The listing builds one solid part. Answer for the finished solid, in the listing's coordinates (mm). A direction names the side the tool comes from. Coordinates: 2 decimals unless noted, no trailing zeros. Order: outer loops, then holes, each group sorted by start corner. A loop starts at its lowest first (then second) coordinate and runs counter-clockwise, first axis right, second up. Notation, with made-up numbers: (21.5, -11.5) -> (62.5, -11.5) arc R11 cw to (62.5, -6.5) -> close; hole circle Ø11 at (68, 71). An arc over 180 degrees is marked (long way). Write each question's results on one line, items separated by ' | '. Start each with the question number.
(1) The part is cut by section C-C, the plane y = -32.5. Give the vertices of the cut face in (x, z), then the cut area to 3 significant figures.
(2) The part is cut by section A-A, the plane y = -14. Give the vertices of the cut face in (x, z).
(3) Determine the mould class of faces 5 (the face through (-7, -50.8, 1)), 6 (the face through (-7, -25, -14.924)), 7 (the face through (-7, -12.471, 28)), 8 (the face through (-7, -7, 39.58)) for opening direction Y: +Y half, -Y half, draft (parallel to the pull), parting line (faces both ways), or undercut.
(4) The part is cut by section D-D, the plane x = -31.5. Give the vertices of the cut face in (y, z), then the cut area to 3 significant figures.
(5) Given pin 1 (10.5 mm diameter, centred on x = -11, y = -33, fed in from +Z); pin 2 (20.5 mm diameter, centred on x = 13.5, z = 31, fed in from -Y), each flat-ended and moving along its own axis, determine where each tip first touches the part or whether it passes through.
(6) A tool of negligible diameter and unlimited length cuts with its end or side. For faces 1 (the face through (-6, -48.26, 2)), 2 (the face through (-49.942, -21, 7)), 3 (the face through (-7, -7, 42.12)), 4 (the face through (-7, -49, 16.72)), from which of +Z, -Z, +X, -X, +Y, -Y can it reach the whole face along a straight path? Write none if from no direction.
(7) The part is cut by section B-B, the plane z = 36. Give the vertices of the cut face in (x, y).
(8) Straight lines are drawn through the part: L1, parallel to Y at x = 11, z = 3.5; L2, parallel to Z at x = -32, y = -12; L3, parallel to Y at x = 7.5, z = 37. For each, find the intervals that lie inside material, in ascending order.
```python
from build123d import *

# Parameters (mm, degrees)
F0_W     = 109.3384288251
F0_H     = 31.6438265145
F1_DEPTH = 50.8
F2_W     = 109.3384288251
F2_H     = 15.0109836832
F3_DEPTH = 25.4
F4_DEPTH = 17.78
F5_T     = -2.54


# Not quite as in the source:
# - a shell that OpenCascade refuses in one call is made with other operations: the cavity is built on its own and cut out


with BuildPart() as f1:
    # F0 (on Front) → F1 (new body)
    with BuildSketch(Plane.XZ):
        with Locations((2.1867696196, 0.8977539837)):
            Rectangle(F0_W, F0_H)
    extrude(amount=F1_DEPTH)

    # F2 (on face) → F3 (join)
    with BuildSketch(Plane.XY.offset(16.719667241)):
        with Locations((2.1867696196, -7.5054918416)):
            Rectangle(F2_W, F2_H)
    extrude(amount=F3_DEPTH)

    # F4 (cut): a face of the model
    f4_faces = [f1.faces().sort_by_distance(p)[0] for p in [
        (56.8559840322, -21.9693633853, 6.3658182119),
    ]]
    extrude(f4_faces, amount=-F4_DEPTH, mode=Mode.SUBTRACT)

    # F5: a shell. OpenCascade refuses it in one call, so the cavity is built on its own and cut out:
    # the body offset inwards by the wall thickness, plus a prism from it out through each open face.
    f5_core = offset(f1.part, amount=F5_T, kind=Kind.INTERSECTION, mode=Mode.PRIVATE)
    f5_exits = [f5_core.faces().sort_by_distance(p)[0] for p in [
        (-6.70323, -30.365492, 14.179667),
    ]]
    add(f5_core, mode=Mode.SUBTRACT)
    extrude(f5_exits, amount=-F5_T, mode=Mode.SUBTRACT)


solid = f1.part
```
Established:
1) outline: (-52.48, -14.92) -> (39.08, -14.92) -> (39.08, 16.72) -> (36.54, 16.72) -> (36.54, -12.38) -> (-49.94, -12.38) -> (-49.94, 16.72) -> (-52.48, 16.72) -> close | area: 380 mm^2
2) outline: (-52.48, -14.92) -> (39.08, -14.92) -> (39.08, 42.12) -> (-52.48, 42.12) -> close; hole (-49.94, -12.38) -> (36.54, -12.38) -> (36.54, 16.72) -> (-49.94, 16.72) -> close
3) face 5: -Y half | face 6: draft | face 7: undercut | face 8: undercut
4) outline: (-50.8, -14.92) -> (0, -14.92) -> (0, 42.12) -> (-15.01, 42.12) -> (-15.01, 16.72) -> (-12.47, 16.72) -> (-12.47, 39.58) -> (-2.54, 39.58) -> (-2.54, -12.38) -> (-48.26, -12.38) -> (-48.26, 16.72) -> (-50.8, 16.72) -> close | area: 431 mm^2
5) pin 1: stops at z = -12.38 | pin 2: stops at y = -15.01
6) face 1: +Z | face 2: none | face 3: +Z, +X, -X, +Y, -Y | face 4: +Z, +X, -X, -Y
7) outline: (-52.48, -15.01) -> (39.08, -15.01) -> (39.08, 0) -> (-52.48, 0) -> close; hole (-49.94, -12.47) -> (36.54, -12.47) -> (36.54, -2.54) -> (-49.94, -2.54) -> close
8) L1: y = -50.8 to -48.26, -2.54 to 0 | L2: z = -14.92 to -12.38, 39.58 to 42.12 | L3: y = -15.01 to -12.47, -2.54 to 0
